Here's how the part is built. I have some questions about the finished solid (model axes, mm). Coordinates: 2 decimals unless noted, no trailing zeros. Write each loop counter-clockwise with the first axis right and the second up, starting at its lowest first coordinate (ties: lowest second). Pieces come first, ordered by that corner, then holes. Notation, with made-up numbers: (89.25, 63.5) -> (130.25, 63.5) arc R23 cw to (130.25, 79.5) -> close; hole circle Ø3 at (22, 10.5). An arc over 180 degrees is marked (long way). Use a Markdown table: item, result. Add a question column.
Item 1: Imagine slicing it at B-B, the plane z = 19.05. Write out the boundary of the cut face in (x, y) (3 decimals).
Item 2: If I drill on line 1 along Y through (x, z) = (-241, 19.05) (3 decimals); line 2 along X through (y, z) = (40, 153); line 3 along Z through (x, y) = (-240.75, 34), over which ranges is the centre line in solid material (lowest first)? Write a range as from..to.
Item 3: Will this pin go through, and if not, where does the flat tip stop? pin 1 Ø5.5 at (y, z) = (34.5, 141.425) entering from +X.
Item 4: Imagine slicing it at A-A, the plane y = 34.5. Write out the boundary of the cut face in (x, z) (3 decimals), and give its area (3 significant figures).
Item 5: Imagine slicing it at C-C, the plane z = 141.5. Count the separate pieces of the cut face and the enclosed holes in it, and give its area (3 significant figures).
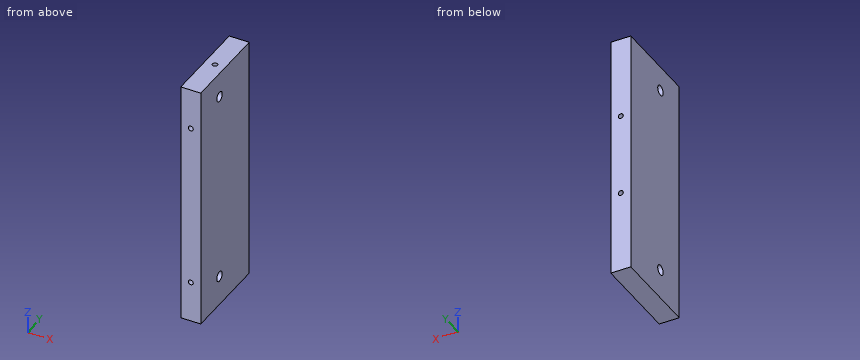
```python
from build123d import *

# Parameters (mm, degrees)
SKETCH1_W                   = 12.7
SKETCH1_H                   = 56.3
BOSS_EXTRUDE1_DEPTH         = 157.3
HOLE1_D                     = 3.175
HOLE1_DEPTH                 = 31.75
HOLE1_CSINK_D               = 10.16
HOLE1_CSINK_ANGLE           = 82
HOLE1_TIP                   = 0.953866233
HOLE2_D                     = 3.175
HOLE2_DEPTH                 = 31.75
HOLE2_CSINK_D               = 10.16
HOLE2_CSINK_ANGLE           = 82
HOLE2_TIP                   = 0.953866233
HOLE_D                      = 3.175
HOLE_DEPTH                  = 31.75
HOLE_CSINK_D                = 10.16
HOLE_CSINK_ANGLE            = 82
HOLE_TIP                    = 0.953866233
HOLE3_D                     = 3.175
HOLE3_DEPTH                 = 31.75
HOLE3_CSINK_D               = 10.16
HOLE3_CSINK_ANGLE           = 82
HOLE3_TIP                   = 0.953866233
HOLE4_D                     = 3.175
HOLE4_DEPTH                 = 31.75
HOLE4_CSINK_D               = 10.16
HOLE4_CSINK_ANGLE           = 82
HOLE4_TIP                   = 0.953866233
F_1_4_0_25_DIAMETER_HOLE1_D = 6.35


with BuildPart() as part:
    # Sketch1 → Boss-Extrude1 (new body)
    with BuildSketch(Plane.XY):
        with Locations((-237.654465963, 40.85)):
            Rectangle(SKETCH1_W, SKETCH1_H)
    extrude(amount=BOSS_EXTRUDE1_DEPTH)

    # Hole1
    with Locations(Plane(origin=(-124.004465969, 0, 2.275709941), x_dir=(1, 0, 0), z_dir=(0, -1, 0))):
        with Locations((113.649999994, 128.807623392), (113.649999994, 23.940956725), (-94.599999994, 161.374290059), (94.599999994, 161.374290059), (0, 161.374290059), (0, 193.124290059), (0, 440.553783621), (0, 301.970350905), (40.979166666, 301.970350905), (166.795833328, 301.970350905), (207.774999994, 440.553783621), (207.774999994, 333.02141023), (207.774999994, 225.48903684), (207.774999994, 137.424290059), (207.774999994, 10.424290059), (-207.774999994, 10.424290059), (-207.774999994, 137.424290059), (-207.774999994, 225.48903684), (-207.774999994, 333.02141023), (-207.774999994, 440.553783621), (-166.795833328, 301.970350905), (-40.979166666, 301.970350905), (-113.649999994, 23.940956725), (-113.649999994, 128.807623392)):
            CounterSinkHole(HOLE1_D / 2, HOLE1_CSINK_D / 2, depth=HOLE1_DEPTH, counter_sink_angle=HOLE1_CSINK_ANGLE)
            with Locations((0, 0, -(HOLE1_DEPTH + HOLE1_TIP / 2))):  # 118° drill point
                Cone(0, HOLE1_D / 2, HOLE1_TIP, mode=Mode.SUBTRACT)

    # Hole2
    with Locations(Plane(origin=(-124.004465969, 0, 155.024290059), x_dir=(-1, 0, 0), z_dir=(0, -1, 0))):
        with Locations((113.649999994, 128.807623392), (113.649999994, 23.940956725), (-94.599999994, 161.374290059), (94.599999994, 161.374290059), (0, 161.374290059), (0, 193.124290059), (0, 440.553783621), (0, 301.970350905), (40.979166666, 301.970350905), (166.795833328, 301.970350905), (207.774999994, 440.553783621), (207.774999994, 333.02141023), (207.774999994, 225.48903684), (207.774999994, 137.424290059), (207.774999994, 10.424290059), (-207.774999994, 10.424290059), (-207.774999994, 137.424290059), (-207.774999994, 225.48903684), (-207.774999994, 333.02141023), (-207.774999994, 440.553783621), (-166.795833328, 301.970350905), (-40.979166666, 301.970350905), (-113.649999994, 23.940956725), (-113.649999994, 128.807623392)):
            CounterSinkHole(HOLE2_D / 2, HOLE2_CSINK_D / 2, depth=HOLE2_DEPTH, counter_sink_angle=HOLE2_CSINK_ANGLE)
            with Locations((0, 0, -(HOLE2_DEPTH + HOLE2_TIP / 2))):  # 118° drill point
                Cone(0, HOLE2_D / 2, HOLE2_TIP, mode=Mode.SUBTRACT)

    # Hole
    with Locations(Plane(origin=(-124.004465969, 277.286738577, 170), x_dir=(-1, 0, 0), z_dir=(0, 0, 1))):
        with Locations((113.649999994, 236.436738577), (207.774999994, 236.436738577)):
            CounterSinkHole(HOLE_D / 2, HOLE_CSINK_D / 2, depth=HOLE_DEPTH, counter_sink_angle=HOLE_CSINK_ANGLE)
            with Locations((0, 0, -(HOLE_DEPTH + HOLE_TIP / 2))):  # 118° drill point
                Cone(0, HOLE_D / 2, HOLE_TIP, mode=Mode.SUBTRACT)

    # Hole3
    with Locations(Plane(origin=(-124.004465969, 88.05, 155.024290059), x_dir=(1, 0, 0), z_dir=(0, 1, 0))):
        with Locations((-162.299999994, -8.625709941), (-113.649999994, 50.157623392), (-113.649999994, 102.590956725), (162.299999994, -8.625709941), (113.649999994, 50.157623392), (113.649999994, 102.590956725), (63.85, 161.374290059), (0, 161.374290059), (-63.85, 161.374290059)):
            CounterSinkHole(HOLE3_D / 2, HOLE3_CSINK_D / 2, depth=HOLE3_DEPTH, counter_sink_angle=HOLE3_CSINK_ANGLE)
            with Locations((0, 0, -(HOLE3_DEPTH + HOLE3_TIP / 2))):  # 118° drill point
                Cone(0, HOLE3_D / 2, HOLE3_TIP, mode=Mode.SUBTRACT)

    # Hole4
    with Locations(Plane(origin=(-124.004465969, 88.05, 2.275709941), x_dir=(-1, 0, 0), z_dir=(0, 1, 0))):
        with Locations((-162.299999994, -8.625709941), (-113.649999994, 50.157623392), (-113.649999994, 102.590956725), (162.299999994, -8.625709941), (113.649999994, 50.157623392), (113.649999994, 102.590956725), (63.85, 161.374290059), (0, 161.374290059), (-63.85, 161.374290059)):
            CounterSinkHole(HOLE4_D / 2, HOLE4_CSINK_D / 2, depth=HOLE4_DEPTH, counter_sink_angle=HOLE4_CSINK_ANGLE)
            with Locations((0, 0, -(HOLE4_DEPTH + HOLE4_TIP / 2))):  # 118° drill point
                Cone(0, HOLE4_D / 2, HOLE4_TIP, mode=Mode.SUBTRACT)

    # 1/4 (0.25) Diameter Hole1 (through all)
    with Locations(Plane.ZY.offset(244.004465963)):
        with Locations((141.425, 34.5), (19.05, 34.5)):
            Hole(F_1_4_0_25_DIAMETER_HOLE1_D / 2)


solid = part.part
```
Ans:
| question | item | result |
|---|---|---|
| 1 | outline | (-244.004, 12.7) -> (-231.304, 12.7) -> (-231.304, 31.325) -> (-244.004, 31.325) -> close; (-244.004, 37.675) -> (-231.304, 37.675) -> (-231.304, 69) -> (-244.004, 69) -> close |
| 2 | line 1 | y = 12.7..31.325, 37.675..69 |
| 2 | line 2 | x = -244..-239, -236.31..-231.3 |
| 2 | line 3 | z = 0..15.91, 22.19..138.29, 144.56..157.3 |
| 3 | pin 1 | passes through |
| 4 | outline | (-244.004, 0) -> (-231.304, 0) -> (-231.304, 15.875) -> (-244.004, 15.875) -> close; (-244.004, 22.225) -> (-231.304, 22.225) -> (-231.304, 138.25) -> (-244.004, 138.25) -> close; (-244.004, 144.6) -> (-231.304, 144.6) -> (-231.304, 157.3) -> (-244.004, 157.3) -> close |
| 4 | area | 1,840 mm^2 |
| 5 | separate pieces | 2 |
| 5 | enclosed holes | 1 |
| 5 | area | 626 mm^2 |
